Work out the finished part from the listing and answer in its coordinate system (mm). A direction names the side the tool comes from. Give positions to 0.01 mm unless a question says otherwise; leave off trailing zeros. Loops run counter-clockwise (first coordinate to the right, second up) from the corner with the lowest first, then second, coordinate; pieces in that order, holes last. Notation, with made-up numbers: (47.5, 65) - (84.5, 65) arc R12 ccw to (84.5, 80) - close; hole circle Ø11 at (8.5, -13.5). An arc over 180 degrees is marked (long way). One line per question, with ' | ' between items. Start each with the question number.
1. Find the intervals of material crossed by line 1 (Z direction, x = 18, y = -68.5); line 2 (Y direction, x = -1.5, z = 5.5); line 3 (Y direction, x = 0.5, z = 13.5), in increasing order.
2. Section D-D (y = -79) is taken. Determine the outline of the cut face in (x, z), plus the area to 3 significant figures.
3. Section A-A (x = 4.5) is taken. Determine the outline of the cut face in (y, z), plus the area to 3 significant figures.
4. Each of these flat-tipped pins is pushed along its axis until it touches: pin 1 (1 mm diameter, centred on x = 6, z = 17, fed in from -Y); pin 2 (1 mm diameter, centred on x = 6.5, z = 13.5, fed in from -Y). Where does it stop, or does it pass through?
5. Section B-B (y = -64) is taken. Determine the outline of the cut face in (x, z), plus the area to 3 significant figures.
6. For a pull along Y with two mould halves and no side action, classify faces 1 (the face through (1, -63, 12.388)), 2 (the face through (19.36, -92.48, -32.54)), 3 (the face through (0.18, -71.95, -32.54)), 4 (the face through (0.18, -71.95, 19.99)) as released by +Y, released by -Y, zero draft, split by the parting line, or undercut.
7. Which of the six approach directions +Z, -Z, +X, -X, +Y, -Y give full straight-line access (tool end or side, diameter ignored) to faces 5 (the face through (1, -49, 27.388)), 6 (the face through (1, -40, -7))?
from build123d import *

# Parameters (mm, degrees)
F0_W     = 50
F0_H     = 65
F1_DEPTH = 40
F2_W     = 50
F2_H     = 15
F3_DEPTH = 60
F4_W     = 50
F4_H     = 10
F5_DEPTH = 60
F6_R     = 24.99999
F7_R     = 10
F8_DEPTH = 92.4


# Not quite as in the source:
# - a fillet or chamfer is up to 0.001 mm smaller than in the source, because OpenCascade refuses the exact size


with BuildPart() as f1:
    # F0 (on Front) → F1 (new body)
    with BuildSketch(Plane.XZ):
        with Locations((1.4840979129, -5.1116640333)):
            Rectangle(F0_W, F0_H)
    extrude(amount=F1_DEPTH)

    # F2 (on face) → F3 (join)
    with BuildSketch(Plane.XZ.offset(40)):
        with Locations((1.4840979129, 19.8883359667)):
            Rectangle(F2_W, F2_H)
    extrude(amount=F3_DEPTH)

    # F4 (on face) → F5 (join)
    with BuildSketch(Plane.XZ.offset(40)):
        with Locations((1.4840979129, -32.6116640333)):
            Rectangle(F4_W, F4_H)
    extrude(amount=F5_DEPTH)

    # F6 (radius 25 in the source; OpenCascade refuses exactly that, so slightly less here)
    f6_edges = [f1.edges().sort_by_distance(p)[0] for p in [
        (-23.515902, -100, -32.611664),
        (-23.515902, -100, 19.888336),
        (26.484098, -100, 19.888336),
        (26.484098, -100, -32.611664),
    ]]
    fillet(f6_edges, radius=F6_R)

    # F7 (on face) → F8 (cut)
    with BuildSketch(Plane.XY.offset(27.3883359667)):
        with Locations((1.4840979129, -81.8661674857)):
            Circle(F7_R)
    extrude(amount=-F8_DEPTH, mode=Mode.SUBTRACT)


solid = f1.part
Conclusion:
1) line 1: -37.61 to -27.61, 12.39 to 27.39 | line 2: -40 to 0 | line 3: -99.98 to -91.82, -71.91 to 0
2) outline: (-23.19, -37.61) - (-8.1, -37.61) - (-8.1, -27.61) - (-23.19, -27.61) - close; (-23.19, 12.39) - (-8.1, 12.39) - (-8.1, 27.39) - (-23.19, 27.39) - close; (11.06, -37.61) - (26.16, -37.61) - (26.16, -27.61) - (11.06, -27.61) - close; (11.06, 12.39) - (26.16, 12.39) - (26.16, 27.39) - (11.06, 27.39) - close | area: 755 mm²
3) outline: (-99.82, -37.61) - (-91.4, -37.61) - (-91.4, -27.61) - (-99.82, -27.61) - close; (-99.82, 12.39) - (-91.4, 12.39) - (-91.4, 27.39) - (-99.82, 27.39) - close; (-72.33, -37.61) - (0, -37.61) - (0, 27.39) - (-72.33, 27.39) - (-72.33, 12.39) - (-40, 12.39) - (-40, -27.61) - (-72.33, -27.61) - close | area: 3,620 mm²
4) pin 1: y = -99.68 | pin 2: y = -99.59
5) outline: (-23.52, -37.61) - (26.48, -37.61) - (26.48, -27.61) - (-23.52, -27.61) - close; (-23.52, 12.39) - (26.48, 12.39) - (26.48, 27.39) - (-23.52, 27.39) - close | area: 1,250 mm²
6) face 1: zero draft | face 2: released by -Y | face 3: undercut | face 4: undercut
7) face 5: +Z, +X, -X, +Y, -Y | face 6: +X, -X, -Y
